```python
from build123d import *

# Parameters (mm, degrees)
F0_W     = 26
F0_H     = 26
F0_W_2   = 22
F0_H_2   = 22
F1_DEPTH = 75
F3_DEPTH = 26.001
F4_R     = 0.5


# Not quite as in the source:
# - a feature names something its author has since deleted; it is built from what else it names


with BuildPart() as f1:
    # F0 (on Top) → F1 (new body)
    with BuildSketch(Plane.XY):
        Rectangle(F0_W, F0_H)
        Rectangle(F0_W_2, F0_H_2, mode=Mode.SUBTRACT)
    extrude(amount=F1_DEPTH)

    # F2 (on face) → F3 (cut, through all)
    with BuildSketch(Plane(origin=(0, 13, 0), x_dir=(-1, 0, 0), z_dir=(0, 1, 0))):
        Polygon((-13, 55.9666790032), (-1.7416697508, 49.4666790032), (10.5, 70.6698729811), (13, 70.6698729811), (13, 75), (-8.7376814767, 75), (-13, 75), align=None)
    extrude(amount=-F3_DEPTH, mode=Mode.SUBTRACT)

    # F4
    f4_edges = [f1.edges().sort_by_distance(p)[0] for p in [
        (13, 13, 27.98334),
        (-13, 13, 35.334936),
        (-13, -13, 35.334936),
        (13, -13, 27.98334),
    ]]
    fillet(f4_edges, radius=F4_R)


solid = f1.part
```
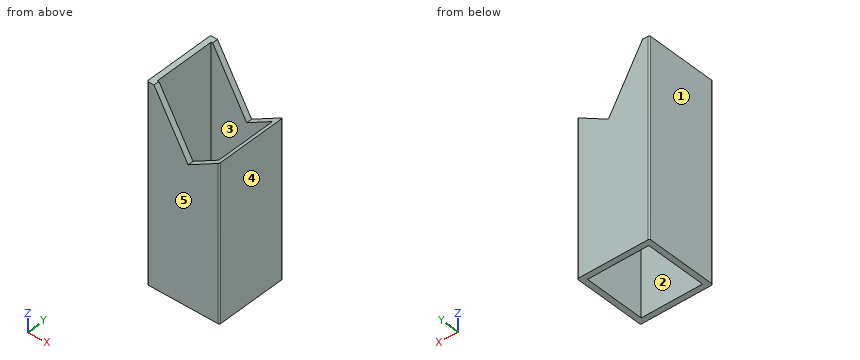
Read the model definition and answer for the solid it produces. Units are mm, in the model's axes. Face numbers are marked on the shaded views. A direction names the side the tool comes from. Round coordinates to 2 decimals unless told otherwise and drop trailing zeros. Write each loop counter-clockwise with the first axis right and the second up, starting at its lowest first coordinate (ties: lowest second). Pieces come first, ordered by that corner, then holes. Notation, with made-up numbers: (62, 45.5) -> (115, 45.5) arc R29 cw to (115, 76.5) -> close; hole circle Ø1 at (73.25, -13.75). An arc over 180 degrees is marked (long way). Answer in a Markdown table with one row per item. Add a question column.
1) Find section C-C, the plane z = 64.5. Determine the outline of the cut face in (x, y), and give its area (3 significant figures).
2) Determine the mould class of the marked faces 3, 4 and 5 for opening direction X: pulls with the +X half, pulls with the -X half, needs draft (parallel to the pull), parting line crosses it, or undercut.
3) Find section B-B, the plane z = 48. Determine the outline of the cut face in (x, y), and give its area (3 significant figures).
4) Consider line 1 (Y direction, x = 6.75, z = 27); line 2 (X direction, y = -4, z = 65). Determine where each line is inside the solid, lowest interval first.
5) Which of the six approach directions +Z, -Z, +X, -X, +Y, -Y give full straight-line access (tool end or side, diameter ignored) to the marked faces 1 and 2?
6) Find section A-A, the plane y = 1.5. Determine the outline of the cut face in (x, z).
Findings below:
| question | item | result |
|---|---|---|
| 1 | outline | (-13, -12.5) arc R0.5 ccw to (-12.5, -13) -> (-6.94, -13) -> (-6.94, -11) -> (-11, -11) -> (-11, 11) -> (-6.94, 11) -> (-6.94, 13) -> (-12.5, 13) arc R0.5 ccw to (-13, 12.5) -> close |
| 1 | area | 68.1 mm² |
| 2 | face 3 | undercut |
| 2 | face 4 | pulls with the +X half |
| 2 | face 5 | needs draft |
| 3 | outline | (-13, -12.5) arc R0.5 ccw to (-12.5, -13) -> (12.5, -13) arc R0.5 ccw to (13, -12.5) -> (13, 12.5) arc R0.5 ccw to (12.5, 13) -> (-12.5, 13) arc R0.5 ccw to (-13, 12.5) -> close; hole (-11, -11) -> (11, -11) -> (11, 11) -> (-11, 11) -> close |
| 3 | area | 192 mm² |
| 4 | line 1 | -13 to -11, 11 to 13 |
| 4 | line 2 | -13 to -11 |
| 5 | face 1 | +Z, -Z, -X, +Y, -Y |
| 5 | face 2 | +Z, -Z |
| 6 | outline | (-13, 0) -> (-11, 0) -> (-11, 70.67) -> (-13, 70.67) -> close; (11, 0) -> (13, 0) -> (13, 55.97) -> (11, 54.81) -> close |
